Model file for the job. Use its own axes, mm. Give positions to 0.01 mm unless a question says otherwise; leave off trailing zeros. Write each loop counter-clockwise with the first axis right and the second up, starting at its lowest first coordinate (ties: lowest second). Pieces come first, ordered by that corner, then holes. Notation, with made-up numbers: (85, 42.25) - (117, 42.25) arc R18 cw to (117, 50.25) - close; hole circle Ø5 at (37.5, 67). An arc over 180 degrees is marked (long way). One line per item, written item: value. Start each with the question number.
(1) Probe L1, parallel to Y at x = 31, z = 8.5; L2, parallel to X at y = -32, z = 10.5. List the from-to ranges inside material, lowest first.
(2) Cut at D-D, the plane x = 114. List the corners of the cut face in (y, z), and give its area (3 significant figures).
(3) Cut at B-B, the plane y = -175. List the corners of the cut face in (x, z).
(4) Cut at A-A, the plane x = 0. List the corners of the cut face in (y, z).
(5) Drop flat-ended pins along their axis: P1, Ø16, axis at x = 0, y = 175, coming from the -Z side; P2, Ø6, axis at x = 29.5, z = 6.5, coming from the +Y side; P3, Ø2, axis at y = 30, z = 4, coming from the -X side; P4, Ø8, axis at y = -189, z = 7.5, coming from the +X side. Give the stop position or say it passes through.
(6) Cut at C-C, the plane z = 5.25. List the corners of the cut face in (x, y).
from build123d import *

# Parameters (mm, degrees)
ESQUISSE1_R             = 245.5
ESQUISSE1_R_2           = 40
BOSS_EXTRU_1_DEPTH      = 15
D_GAGEMENT_M20_D        = 17.5
D_GAGEMENT_M20_DEPTH    = 15
CHANFREIN1_SIZE         = 2
ENL_V_MAT_EXTRU_1_REACH = 17
ESQUISSE4_R             = 7.5


with BuildPart() as part:
    # Esquisse1 → Boss.-Extru.1 (new body)
    with BuildSketch(Plane.XY):
        Circle(ESQUISSE1_R)
        Circle(ESQUISSE1_R_2, mode=Mode.SUBTRACT)
    extrude(amount=BOSS_EXTRU_1_DEPTH)

    # Dégagement M20
    with Locations(Plane.XY.offset(15)):
        with Locations((0, 175), (0, -175)):
            Hole(D_GAGEMENT_M20_D / 2, depth=D_GAGEMENT_M20_DEPTH)

    # Chanfrein1
    chanfrein1_edges = [part.edges().sort_by_distance(p)[0] for p in [
        (-40, 0, 0),
        (-40, 0, 15),
    ]]
    chamfer(chanfrein1_edges, length=CHANFREIN1_SIZE)

    # Esquisse4 → Enlèv. mat.-Extru.1 (cut, up to next)
    with BuildSketch(Plane(origin=(0, 0, 0), x_dir=(-1, 0, 0), z_dir=(0, 0, -1)), mode=Mode.PRIVATE) as enl_v_mat_extru_1_sk1:
        with Locations((0, -245.5)):
            Circle(ESQUISSE4_R)
    enl_v_mat_extru_1_tool1 = extrude(enl_v_mat_extru_1_sk1.sketch, amount=-ENL_V_MAT_EXTRU_1_REACH, mode=Mode.PRIVATE) & part.part
    add(enl_v_mat_extru_1_tool1.solids().sort_by_distance((0, -245.5, 0))[0], mode=Mode.SUBTRACT)


solid = part.part
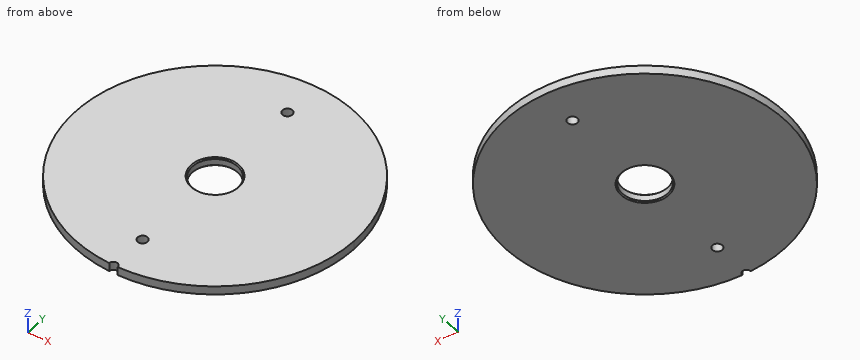
Answers follow:
1. L1: y = -243.53 to -25.28, 25.28 to 243.53
1. L2: x = -243.41 to -24, 24 to 243.41
2. outline: (-217.43, 0) - (217.43, 0) - (217.43, 15) - (-217.43, 15) - close
2. area: 6,520 mm²
3. outline: (-172.18, 0) - (-8.75, 0) - (-8.75, 15) - (-172.18, 15) - close; (8.75, 0) - (172.18, 0) - (172.18, 15) - (8.75, 15) - close
4. outline: (-238, 0) - (-183.75, 0) - (-183.75, 15) - (-238, 15) - close; (-166.25, 0) - (-42, 0) - (-40, 2) - (-40, 13) - (-42, 15) - (-166.25, 15) - close; (40, 2) - (42, 0) - (166.25, 0) - (166.25, 15) - (42, 15) - (40, 13) - close; (183.75, 0) - (245.5, 0) - (245.5, 15) - (183.75, 15) - close
5. P1: passes through
5. P2: stops at y = 244.07
5. P3: stops at x = -243.78
5. P4: stops at x = 161.39
6. outline: (-7.5, -245.39) arc R7.5 cw to (7.5, -245.39) arc R245.5 ccw (long way) to start; hole circle Ø80 at (0, 0); hole circle Ø17.5 at (0, -175); hole circle Ø17.5 at (0, 175)
